Input: part model. Units: mm. Frame: model coordinates. A direction names the side the tool comes from. Coordinates: 2 decimals unless noted, no trailing zeros. Loops run counter-clockwise (first coordinate to the right, second up) from the corner with the lowest first, then second, coordinate; pieces in that order, holes last. Notation, with made-up numbers: (2, 41) - (30, 41) arc R31 cw to (30, 79) - close; hole circle Ø1 at (-29, 21.5). An arc over 180 degrees is marked (long way). Use a Markdown table: item, result. Add a question column.
1. Section query A-A on x = 29. Return the cut outline in (y, z), then the cut area to 3 significant figures.
2. Ray query, L1, parallel to X at y = 9.75, z = 2; L2, parallel to Y at x = 72, z = 2.5; L3, parallel to X at y = 10, z = -0.25. Return the intervals inside material, ascending. Write a range as [from, to].
3. Section query B-B on z = -1.5. Return the cut outline in (x, y).
4. Contact query for flat-ended pins moving along their axis: P1, Ø1.5, axis at y = 8.5, z = -0.5, coming from the +X side; P2, Ø1.5, axis at x = 102.5, z = -1.5, coming from the -Y side; P3, Ø8, axis at x = 59, y = 2.5, coming from the -Z side; P4, Ø2.5, axis at x = 22.5, z = -2, coming from the +Y side. Output: stop coordinate, or through.
5. Access query for faces 5 (the face through (102, 12.75, -1)), 6 (the face through (25.6, 15.43, 2.03)), 7 (the face through (118, 10, 3.8)), 8 (the face through (23, 7.25, -1)). Directions: +Z, -Z, +X, -X, +Y, -Y. A direction counts if a zero-diameter tool reaches every point of the face in a straight line with its end or side. Return the directions, or none.
6. Draft query along Y for faces 1 (the face through (12, 16, 2)), 2 (the face through (100, 10, 0)), 3 (the face through (0.57, 19.4, 1.97)), 4 (the face through (62, 0, 2)). Return one class per face: released by +Y, released by -Y, zero draft, split by the parting line, or undercut.
Autodesk Fusion 360 part; units mm, degrees
sketch "Sketch1" plane through (0, 0, 0) normal (0, 0, 1) x (1, 0, 0)
  line L0 (2, 0) -> (123, 0)
  line L1 (125, 2) -> (125, 18)
  line L2 (123, 20) -> (2, 20)
  line L3 (0, 18) -> (0, 2)
  arc A0 (2, 20) -> (0, 18) centre (2, 18) ccw
  arc A1 (0, 2) -> (2, 0) centre (2, 2) ccw
  arc A2 (123, 0) -> (125, 2) centre (123, 2) ccw
  arc A3 (125, 18) -> (123, 20) centre (123, 18) ccw
  line L4 (4, 4) -> (121, 4)
  line L5 (121, 4) -> (121, 16)
  line L6 (121, 16) -> (4, 16)
  line L7 (4, 16) -> (4, 4)
  line L8 (20, 16) -> (25, 16)
  line L9 (25, 16) -> (25, 4)
  line L10 (25, 4) -> (20, 4)
  line L11 (20, 4) -> (20, 16)
  line L12 (62.5, 0) -> (62.5, 20) construction
  line L13 (105, 4) -> (105, 16)
  line L14 (105, 16) -> (100, 16)
  line L15 (100, 4) -> (105, 4)
  line L16 (100, 16) -> (100, 4)
  line L17 (20, 12.75) -> (105, 12.75)
  line L18 (105, 12.75) -> (105, 7.25)
  line L19 (105, 7.25) -> (20, 7.25)
  line L20 (20, 7.25) -> (20, 12.75)
  line L21 (20, 12.75) -> (105, 7.25) construction
  line L22 (105, 12.75) -> (20, 7.25) construction
  line L23 (9, 16) -> (9, 4)
  line L24 (116, 16) -> (116, 4)
  point P0 (125, 0)
  point P1 (0, 20)
  point P2 (62.5, 10)
  dimension "d1" = 125
  dimension "d2" = 20
  dimension "d3" = 2
  dimension "d4" = -4
  dimension "d5" = 5
  dimension "d7" = 80
  dimension "d16" = 5.5
  dimension "d23" = 5
  dimension "d24" = 5
extrude "Extrude1" add sketch "Sketch1" along normal blind 4 contours L0 L1 L2 L3 A0 A1 A2 A3 | L4 L9 L10 L11 L19 | L9 L11 L17 L19 L20 | L6 L8 L9 L11 L17 | L4 L13 L15 L16 L19 | L13 L16 L17 L18 L19 | L6 L13 L14 L16 L17
extrude "Extrude3" add sketch "Sketch1" against normal blind 4 contours L9 L11 L17 L19 L20 | L13 L16 L17 L18 L19
extrude "Extrude4" add sketch "Sketch1" against normal blind 0.2 from surface at 4 contours L4 L6 L7 L23 | L4 L5 L6 L24
fillet "Fillet1" radius 1 4 edges at (22.5, 12.75, -4) (22.5, 7.25, -4) (102.5, 12.75, -4) (102.5, 7.25, -4)
fillet "Fillet2" radius 2 12 edges at (121, 4, 2) (105, 4, 2) (100, 4, 2) (121, 16, 2) (105, 16, 2) (100, 16, 2) (20, 4, 2) (4, 4, 2) (4, 16, 2) (20, 16, 2) (25, 4, 2) (25, 16, 2)
Resolved:
| question | item | result |
|---|---|---|
| 1 | outline | (0, 0) - (4, 0) - (4, 4) - (0, 4) - close; (16, 0) - (20, 0) - (20, 4) - (16, 4) - close |
| 1 | area | 32.0 mm² |
| 2 | L1 | [0, 4], [20, 25], [100, 105], [121, 125] |
| 2 | L2 | [0, 4], [16, 20] |
| 2 | L3 | [20, 25], [100, 105] |
| 3 | outline | (20, 7.25) - (25, 7.25) - (25, 12.75) - (20, 12.75) - close; (100, 7.25) - (105, 7.25) - (105, 12.75) - (100, 12.75) - close |
| 4 | P1 | x = 125 |
| 4 | P2 | y = 7.25 |
| 4 | P3 | z = 0 |
| 4 | P4 | y = 12.75 |
| 5 | face 5 | -Z, +X, -X, +Y |
| 5 | face 6 | +Z, -Z |
| 5 | face 7 | -Z |
| 5 | face 8 | -Z, +X, -X, -Y |
| 6 | face 1 | undercut |
| 6 | face 2 | undercut |
| 6 | face 3 | released by +Y |
| 6 | face 4 | released by -Y |
